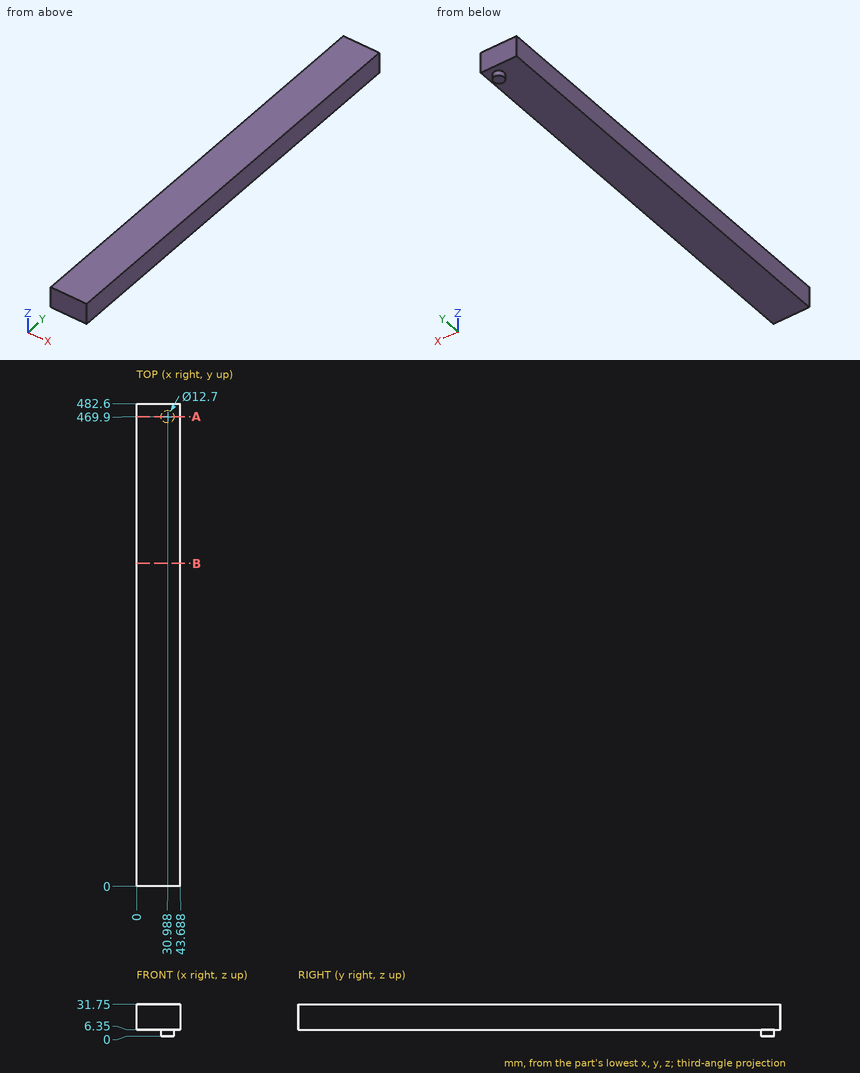
Geometry check sheet. Reference: drawing and pictorial views, mm from the part's lowest x, y, z. Coordinates: 2 decimals unless noted, no trailing zeros. Order: outer loops, then holes, each group sorted by start corner. A loop starts at its lowest first (then second) coordinate and runs counter-clockwise, first axis right, second up.
Item 1: Depth check by flat-ended pin: pin 1 (3 mm diameter, centred on x = 37, z = 16.5, fed in from -Y); pin 2 (12 mm diameter, centred on x = 16.5, y = 56, fed in from -Z). Enter the tip coordinate at first touch or a pass-through.
Item 2: Section check A-A (y = 469.9). Enter the section's corners in (x, z).
Item 3: Scan line: line 1 along Z through (x, y) = (15, 323). Record every from-to range of solid material in increasing order.
Item 4: Section check B-B (y = 323). Enter the section's corners in (x, z), plus the area to 3 significant figures.
Check sheet entries:
1. pin 1: stops at y = 0
1. pin 2: stops at z = 6.35
2. outline: (0, 6.35) - (24.64, 6.35) - (24.64, 0) - (37.34, 0) - (37.34, 6.35) - (43.69, 6.35) - (43.69, 31.75) - (0, 31.75) - close
3. line 1: z = 6.35 to 31.75
4. outline: (0, 6.35) - (43.69, 6.35) - (43.69, 31.75) - (0, 31.75) - close
4. area: 1,110 mm2
